Can you work these out from the drawing? Everything is in mm from the part's minimum corner. Give positions to 0.01 mm unless a question says otherwise; leave off trailing zeros. Loops run counter-clockwise (first coordinate to the right, second up) from the corner with the lowest first, then second, coordinate; pieces in that order, holes last.
Q1. If we section it at D-D (z = 21.25): Please give me the cut outline in (x, y), plus the area to 3 significant figures.
Q2. If we section it at A-A (x = 90): Please give me the cut outline in (y, z), plus the area to 3 significant figures.
Q3. If we section it at C-C (z = 10): Please give me the cut outline in (x, y), plus the area to 3 significant figures.
Q4. I need wall thicknesses on line 1 (X direction, y = 3.5, z = 10); line 2 (Z direction, x = 67, y = 6). Which ranges of each line are inside material? Lowest first, please.
Q5. If we section it at B-B (y = 4.5): Please give me the cut outline in (x, z).
Q6. Will these pins go through, and if not, where does the flat tip stop? P1, Ø4.5, axis at x = 10, z = 10, coming from the +Y side; P2, Ø1.9, axis at y = 2, z = 23.5, coming from the -X side.
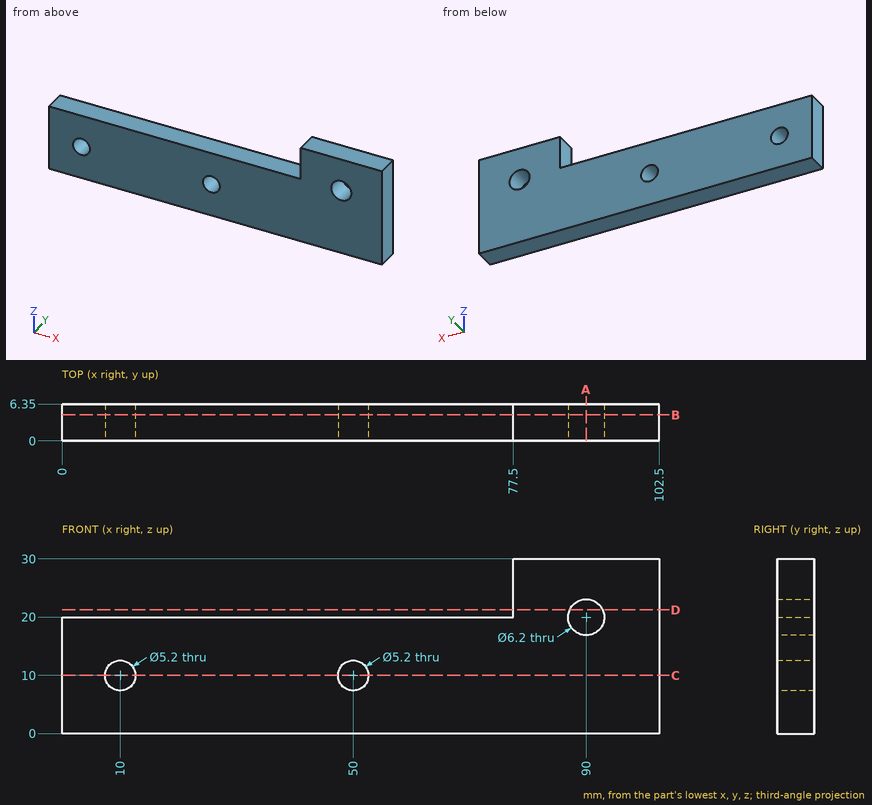
Check sheet entries:
1. outline: (77.5, 0) - (87.16, 0) - (87.16, 6.35) - (77.5, 6.35) - close; (92.84, 0) - (102.5, 0) - (102.5, 6.35) - (92.84, 6.35) - close
1. area: 123 mm2
2. outline: (0, 0) - (6.35, 0) - (6.35, 16.9) - (0, 16.9) - close; (0, 23.1) - (6.35, 23.1) - (6.35, 30) - (0, 30) - close
2. area: 151 mm2
3. outline: (0, 0) - (7.4, 0) - (7.4, 6.35) - (0, 6.35) - close; (12.6, 0) - (47.4, 0) - (47.4, 6.35) - (12.6, 6.35) - close; (52.6, 0) - (102.5, 0) - (102.5, 6.35) - (52.6, 6.35) - close
3. area: 585 mm2
4. line 1: x = 0 to 7.4, 12.6 to 47.4, 52.6 to 102.5
4. line 2: z = 0 to 20
5. outline: (0, 0) - (102.5, 0) - (102.5, 30) - (77.5, 30) - (77.5, 20) - (0, 20) - close; hole circle Ø5.2 at (10, 10); hole circle Ø5.2 at (50, 10); hole circle Ø6.2 at (90, 20)
6. P1: passes through
6. P2: stops at x = 77.5
